from build123d import *

# Parameters (mm, degrees)
RESSALTO_EXTRUS_O1_DEPTH                   = 12
RESSALTO_EXTRUS_O1_DEPTH_BACK              = 12
ESBO_O1_W                                  = 75
ESBO_O1_H                                  = 70
ESBO_O3_R                                  = 5.5
CORTE_EXTRUS_O1_DEPTH                      = 525.799189678
ESBO_O4_R                                  = 4.1
CORTE_EXTRUS_O2_DEPTH                      = 20
FILETE1_R                                  = 2
CORTE_EXTRUS_O3_DEPTH                      = 29
CORTE_EXTRUS_O4_DEPTH                      = 28
RESSALTO_EXTRUS_O2_DEPTH                   = 6
RESSALTO_EXTRUS_O2_DEPTH_BACK              = 30
ESBO_O7_W                                  = 7
ESBO_O7_H                                  = 8
BROCA_DE_ROSQUEAR_PARA_TARRAXA_DE_M2X0_4_D = 1.6
BROCA_DE_ROSQUEAR_PARA_TARRAXA_DE_M2_2_D   = 1.6
ESBO_O18_W                                 = 20
ESBO_O18_H                                 = 4
RESSALTO_EXTRUS_O3_DEPTH                   = 10


with BuildPart() as part:
    # Esbo_o1 → Ressalto-extrus_o1 (new, two sides: drawn at the far end of the back side and taken through both)
    with BuildSketch(Plane(origin=(-220, 0, 0), x_dir=(0, 0, -1), z_dir=(1, 0, 0)).offset(-RESSALTO_EXTRUS_O1_DEPTH_BACK)):
        with Locations((-427.999935002, 213.253952806)):
            Rectangle(ESBO_O1_W, ESBO_O1_H)
    extrude(amount=RESSALTO_EXTRUS_O1_DEPTH + RESSALTO_EXTRUS_O1_DEPTH_BACK)

    # Esbo_o3 → Corte-extrus_o1 (cut, through all)
    with BuildSketch(Plane(origin=(0, 248.253952806, 0), x_dir=(1, 0, 0), z_dir=(0, 1, 0))):
        with Locations(Location((-219.508549322, -425.149935105, 0), (0, 0, 270))):
            Circle(ESBO_O3_R)
        with BuildLine():
            Line((-220, -465.499935002), (-218, -465.499935002))
            Line((-218, -465.499935002), (-218, -460.369179456))
            ThreePointArc((-218, -460.369179456), (-219.711945476, -445.401349285), (-222, -460.292000844))
            Line((-222, -460.292000844), (-222, -465.499935002))
            Line((-222, -465.499935002), (-220, -465.499935002))
        make_face()
    extrude(amount=-CORTE_EXTRUS_O1_DEPTH, mode=Mode.SUBTRACT)

    # Esbo_o4 → Corte-extrus_o2 (cut)
    with BuildSketch(Plane(origin=(0, 0, 390.499935002), x_dir=(-1, 0, 0), z_dir=(0, 0, -1))):
        with Locations(Location((219.858557552, 238.253952806, 0), (0, 0, 90))):
            Circle(ESBO_O4_R)
        with Locations(Location((219.858557552, 188.253952806, 0), (0, 0, 90))):
            Circle(ESBO_O4_R)
    extrude(amount=-CORTE_EXTRUS_O2_DEPTH, mode=Mode.SUBTRACT)

    # Filete1
    filete1_edges = [part.edges().sort_by_distance(p)[0] for p in [
        (-208, 213.253952806, 465.499935002),
        (-232, 213.253952806, 390.499935002),
        (-208, 178.253952806, 427.999935002),
        (-208, 213.253952806, 390.499935002),
        (-208, 248.253952806, 427.999935002),
        (-232, 248.253952806, 427.999935002),
        (-213, 178.253952806, 465.499935002),
        (-213, 248.253952806, 465.499935002),
        (-232, 213.253952806, 465.499935002),
        (-227, 248.253952806, 465.499935002),
        (-220, 248.253952806, 390.499935002),
        (-220, 178.253952806, 390.499935002),
        (-227, 178.253952806, 465.499935002),
        (-232, 178.253952806, 427.999935002),
    ]]
    fillet(filete1_edges, radius=FILETE1_R)

    # Esbo_o5 → Corte-extrus_o3 (cut)
    with BuildSketch(Plane(origin=(0, 0, 390.499935002), x_dir=(-1, 0, 0), z_dir=(0, 0, -1))):
        Polygon((214.029355297, 195.258459884), (226.029351267, 195.248625677), (226.058853888, 231.248613588), (214.058857917, 231.258447795), align=None)
    extrude(amount=-CORTE_EXTRUS_O3_DEPTH, mode=Mode.SUBTRACT)

    # Esbo_o6 → Corte-extrus_o4 (cut)
    with BuildSketch(Plane.ZY.offset(232)):
        with BuildLine():
            Line((399.499935002, 215.753952806), (412.499935002, 215.753952806))
            ThreePointArc((412.499935002, 215.753952806), (413.207041783, 215.461059587), (413.499935002, 214.753952806))
            Line((413.499935002, 214.753952806), (413.499935002, 211.753952806))
            ThreePointArc((413.499935002, 211.753952806), (413.207041783, 211.046846025), (412.499935002, 210.753952806))
            Line((412.499935002, 210.753952806), (399.499935002, 210.753952806))
            ThreePointArc((399.499935002, 210.753952806), (398.792828221, 211.046846025), (398.499935002, 211.753952806))
            Line((398.499935002, 211.753952806), (398.499935002, 214.753952806))
            ThreePointArc((398.499935002, 214.753952806), (398.792828221, 215.461059587), (399.499935002, 215.753952806))
        make_face()
    extrude(amount=-CORTE_EXTRUS_O4_DEPTH, mode=Mode.SUBTRACT)

    # Esbo_o7 → Ressalto-extrus_o2 (add, two sides: drawn at the far end of the back side and taken through both)
    with BuildSketch(Plane(origin=(-208, 0, 0), x_dir=(0, 0, -1), z_dir=(1, 0, 0)).offset(-RESSALTO_EXTRUS_O2_DEPTH_BACK)):
        with Locations((-441.999935002, 213.253952806)):
            Rectangle(ESBO_O7_W, ESBO_O7_H)
    extrude(amount=RESSALTO_EXTRUS_O2_DEPTH + RESSALTO_EXTRUS_O2_DEPTH_BACK)

    # Broca de rosquear para tarraxa de M2x0.4 (through all)
    with Locations(Plane.XY.offset(445.499935002)):
        with Locations((-205, 213.253952806)):
            Hole(BROCA_DE_ROSQUEAR_PARA_TARRAXA_DE_M2X0_4_D / 2)

    # Broca de rosquear para tarraxa de M2 2 (through all)
    with Locations(Plane.XY.offset(445.499935002)):
        with Locations((-235, 213.253952806)):
            Hole(BROCA_DE_ROSQUEAR_PARA_TARRAXA_DE_M2_2_D / 2)

    # Esbo_o18 → Ressalto-extrus_o3 (add)
    with BuildSketch(Plane(origin=(0, 248.253952806, 0), x_dir=(1, 0, 0), z_dir=(0, 1, 0))):
        with Locations((-220, -398.434558943)):
            Rectangle(ESBO_O18_W, ESBO_O18_H)
    extrude(amount=RESSALTO_EXTRUS_O3_DEPTH)


solid = part.part
Work out the finished part from the listing and answer in its coordinate system (mm). A direction names the side the tool comes from. Round coordinates to 2 decimals unless told otherwise and drop trailing zeros. Write each loop counter-clockwise with the first axis right and the second up, starting at its lowest first coordinate (ties: lowest second). Pieces come first, ordered by that corner, then holes. Notation, with made-up numbers: M 12.25,-30 L 35.25,-30 A15 cw 35.25,-3 Z; hole C -0.75,-28.75 d5. An arc over 180 degrees is marked long. Use a Markdown table: item, result.
1) The part is cut by section A-A on z = 418. Give the vertices of the cut face in (x, y), plus the area to 3 significant figures.
Taken from the geometry:
| item | result |
|---|---|
| outline | M -232,180.25 A2 ccw -230,178.25 L -210,178.25 A2 ccw -208,180.25 L -208,246.25 A2 ccw -210,248.25 L -230,248.25 A2 ccw -232,246.25 Z; hole M -226.06,231.25 L -226.03,195.25 L -214.03,195.26 L -214.06,231.26 Z |
| area | 1,240 mm2 |
2) Flat-ended cylindrical pins translate along their axes: pin 1 (3 mm diameter, centred on x = -205.5, z = 443, fed in from -Y); pin 2 (10 mm diameter, centred on y = 243, z = 414.5, fed in from -X); pin 3 (8 mm diameter, centred on x = -207, z = 433, fed in from +Y). Find the tip coordinate at first contact, or state that the pin passes through.
Taken from the geometry:
| item | result |
|---|---|
| pin 1 | stops at y = 209.25 |
| pin 2 | stops at x = -232 |
| pin 3 | stops at y = 248.25 |
3) The part is cut by section C-C on y = 250.5. Give the vertices of the cut face in (x, z).
Taken from the geometry:
| item | result |
|---|---|
| outline | M -230,396.43 L -210,396.43 L -210,400.43 L -230,400.43 Z |
4) Consider line 1 (X direction, y = 220.5, z = 410); line 2 (Y direction, x = -210, z = 410.5); line 3 (Z direction, x = -220, y = 210). Determine where each line is inside the solid, lowest interval first. Write a range as [from, to].
Taken from the geometry:
| item | result |
|---|---|
| line 1 | x = [-232, -226.05], [-214.05, -208] |
| line 2 | y = [178.25, 210.75], [215.75, 248.25] |
| line 3 | z = [419.5, 419.67], [430.63, 445.5] |
5) Determine the mould class of faces 4 (the face through (-225.94, 247.65, 464.93)), 5 (the face through (-205, 209.254, 442)), 6 (the face through (-224.02, 213.74, 446.64)) for opening direction Z: pulls with the +Z half, pulls with the -Z half, needs draft (parallel to the pull), parting line crosses it, or undercut.
Taken from the geometry:
| item | result |
|---|---|
| face 4 | pulls with the +Z half |
| face 5 | needs draft |
| face 6 | undercut |
6) Which of the six approach directions +Z, -Z, +X, -X, +Y, -Y give full straight-line access (tool end or side, diameter ignored) to faces 1 (the face through (-220, 213, 445.5)), 2 (the face through (-229, 210.754, 406)), 3 (the face through (-235, 212, 438.5))?
Taken from the geometry:
| item | result |
|---|---|
| face 1 | +Z, +Y, -Y |
| face 2 | +X, -X |
| face 3 | -Z, -X, +Y, -Y |
7) The part is cut by section B-B on y = 232.5. Give the vertices of the cut face in (x, z).
Taken from the geometry:
| item | result |
|---|---|
| outline | M -232,392.5 A2 ccw -230,390.5 L -210,390.5 A2 ccw -208,392.5 L -208,463.5 A2 ccw -210,465.5 L -218,465.5 L -218,460.37 A7.6 cw long -222,460.29 L -222,465.5 L -230,465.5 A2 ccw -232,463.5 Z; hole C -219.51,425.15 d11 |
